The listing builds one solid part. Answer for the finished solid, in the listing's coordinates (mm). Face numbers are marked on the shaded views. A direction names the side the tool comes from. Coordinates: 2 decimals unless noted, no trailing zeros. Order: outer loops, then holes, each group sorted by start corner. A loop starts at its lowest first (then second) coordinate and runs counter-clockwise, first axis right, second up.
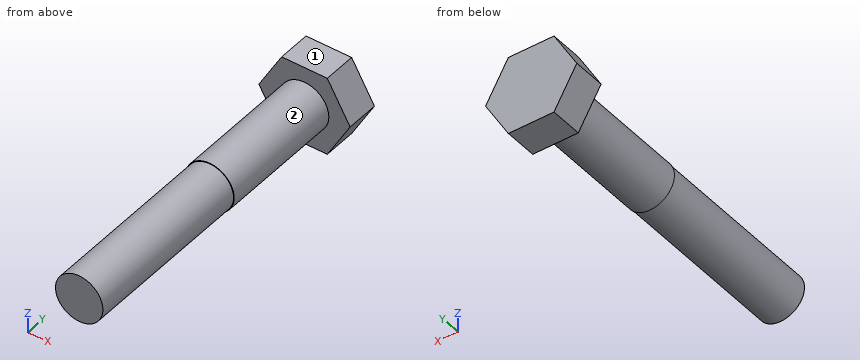
```python
from build123d import *

# Parameters (mm, degrees)
F0_R     = 4
F1_DEPTH = 50
F2_DEPTH = 5.4
F3_R     = 4
F3_R_2   = 3.9
F4_DEPTH = 29


with BuildPart() as f1:
    # F0 (on Front) → F1 (new body)
    with BuildSketch(Plane.XZ):
        Circle(F0_R)
    extrude(amount=F1_DEPTH)

    # F0 (on Front) → F2 (join)
    with BuildSketch(Plane.XZ):
        Polygon((3.7527767497, 6.5), (-3.7527767497, 6.5), (-7.5055534995, 0), (-3.7527767497, -6.5), (3.7527767497, -6.5), (7.5055534995, 0), align=None)
        Circle(F0_R, mode=Mode.SUBTRACT)
        Circle(F0_R)
    extrude(amount=-F2_DEPTH)

    # F3 (on face) → F4 (cut)
    with BuildSketch(Plane.XZ.offset(50)):
        Circle(F3_R)
        Circle(F3_R_2, mode=Mode.SUBTRACT)
    extrude(amount=-F4_DEPTH, mode=Mode.SUBTRACT)


solid = f1.part
```
(1) Find section B-B (y = -42). Write down the section's boundary in (x, z).
(2) This flat-tipped pin is pushed along its axis until it touches: pin 1 Ø2 at (x, y) = (4, -28.5) entering from -Z. Where does it stop, or does it pass through?
(3) Find section C-C (z = -0.75). Write down the section's boundary in (x, y).
(4) For the marked faces 1 and 2, determine the directions among +Z, -Z, +X, -X, +Y, -Y from which every point of the face is accessible in a straight line to the end or side of a thin tool.
(5) Find section A-A (x = 0). Write down the section's boundary in (y, z), and give its area (3 significant figures).
(6) Find section D-D (x = 4.75). Write down the section's boundary in (y, z).
(7) Consider line 1 (Y direction, x = 4.5, z = 4.75); line 2 (Z direction, x = 0, y = -0.5); line 3 (Z direction, x = 2.25, y = -24.5). Determine where each line is inside the solid, lowest interval first.
Findings below:
1. outline: circle Ø7.8 at (0, 0)
2. pin 1: stops at z = -2.49
3. outline: (-7.07, 0) - (-3.93, 0) - (-3.93, -21) - (-3.83, -21) - (-3.83, -50) - (3.83, -50) - (3.83, -21) - (3.93, -21) - (3.93, 0) - (7.07, 0) - (7.07, 5.4) - (-7.07, 5.4) - close
4. face 1: +Z, +X, -X, +Y, -Y
4. face 2: -Y
5. outline: (-50, -3.9) - (-21, -3.9) - (-21, -4) - (0, -4) - (0, -6.5) - (5.4, -6.5) - (5.4, 6.5) - (0, 6.5) - (0, 4) - (-21, 4) - (-21, 3.9) - (-50, 3.9) - close
5. area: 464 mm2
6. outline: (0, -4.77) - (5.4, -4.77) - (5.4, 4.77) - (0, 4.77) - close
7. line 1: y = 0 to 5.4
7. line 2: z = -4 to 4
7. line 3: z = -3.19 to 3.19
